from build123d import *

# Parameters (mm, degrees)
F0_W      = 12.5
F0_H      = 13.2
F1_DEPTH  = 6.5
F2_R      = 3.5
F3_DEPTH  = 5
F4_R      = 3
F5_DEPTH  = 10
F6_SIZE   = 0.5
F7_W      = 12.7
F7_H      = 1.5
F8_DEPTH  = 7
F10_DEPTH = 1


with BuildPart() as f1:
    # F0 (on Top) → F1 (new body)
    with BuildSketch(Plane.XY):
        Rectangle(F0_W, F0_H)
    extrude(amount=F1_DEPTH)

    # F2 (on face) → F3 (join)
    with BuildSketch(Plane.XY.offset(6.5)):
        Circle(F2_R)
    extrude(amount=F3_DEPTH)

    # F4 (on face) → F5 (join)
    with BuildSketch(Plane.XY.offset(11.5)):
        Circle(F4_R)
    extrude(amount=F5_DEPTH)

    # F6
    f6_edges = [f1.edges().sort_by_distance(p)[0] for p in [
        (-3, 0, 21.5),
    ]]
    chamfer(f6_edges, length=F6_SIZE)

    # F7 (on face) → F8 (cut)
    with BuildSketch(Plane.XY.offset(21.5)):
        with Locations((0, -2.25)):
            Rectangle(F7_W, F7_H)
    extrude(amount=-F8_DEPTH, mode=Mode.SUBTRACT)

    # F9 (on Front) → F10 (join, symmetric)
    with BuildSketch(Plane.XZ):
        Polygon((-6.25, 3.25), (-7, 3.25), (-7, -3.5), (-6.5, -3.5), (-6.5, 2.75), (-6.25, 2.75), align=None)
        Polygon((6.25, 2.75), (6.5, 2.75), (6.5, -3.5), (7, -3.5), (7, 3.25), (6.25, 3.25), align=None)
    extrude(amount=F10_DEPTH, both=True)


solid = f1.part
Geometry check sheet. Reference: the model listing, model coordinates, mm. A direction names the side the tool comes from. Round coordinates to 2 decimals unless told otherwise and drop trailing zeros. Loops run counter-clockwise (first coordinate to the right, second up) from the corner with the lowest first, then second, coordinate; pieces in that order, holes last. Notation, with made-up numbers: (31.25, 48.5) - (64.25, 48.5) arc R16 cw to (64.25, 77.5) - close; hole circle Ø10 at (48.25, -2.5). An arc over 180 degrees is marked (long way). One line per question, with ' | ' between items. Start each with the question number.
1. Tool access check on faces 5 (the face through (0, -2, 14.5)), 6 (the face through (0, 6.6, 3)), 7 (the face through (1.61, 2.53, 16.18)). Record the directions out of +Z, -Z, +X, -X, +Y, -Y that give a thin tool (end or side, any length) a straight path to the whole face; none if there is none.
2. Cross-section at D-D on z = 16.25. Record the cut outline in (x, y).
3. Cross-section at A-A on z = -1.25. Record the cut outline in (x, y), then the cut area to 3 significant figures.
4. Depth check by flat-ended pin: pin 1 (4 mm diameter, centred on x = -1.5, y = 0, fed in from -Z); pin 2 (0.8 mm diameter, centred on x = -7, y = 0, fed in from +Z); pin 3 (0.6 mm diameter, centred on x = -6.5, z = -1, fed in from -Y). Enter the tip coordinate at first touch or a pass-through.
5. Scan lines: line 1 (X direction, y = 1.5, z = 4.5); line 2 (Z direction, x = 6, y = -5); line 3 (Z direction, x = 1.25, y = 1.25). Record each from-to range of solid material in increasing order. Write a range as [from, to].
6. Draft check along X on faces 1 (the face through (-6.5, 0, 0)), 2 (the face through (0.082, 2.634, 21.365)), 3 (the face through (0, -6.6, 3)), 4 (the face through (6.5, 0, 0)). Enter one of: released by +X, released by -X, zero draft, split by the parting line, or undercut.
7. Cross-section at C-C on x = 0. Record the cut outline in (y, z), then the cut area to 3 significant figures.
8. Cross-section at B-B on y = 0. Record the cut outline in (x, z), then the cut area to 3 significant figures.
Taken from the geometry:
1) face 5: +Z, +X, -X, -Y | face 6: +Z, -Z, +X, -X, +Y | face 7: +Z
2) outline: (-2.6, -1.5) - (2.6, -1.5) arc R3 ccw (long way) to start
3) outline: (-7, -1) - (-6.5, -1) - (-6.5, 1) - (-7, 1) - close; (6.5, -1) - (7, -1) - (7, 1) - (6.5, 1) - close | area: 2.00 mm²
4) pin 1: z = 0 | pin 2: z = 3.25 | pin 3: y = -1
5) line 1: [-6.25, 6.25] | line 2: [0, 6.5] | line 3: [0, 21.5]
6) face 1: undercut | face 2: split by the parting line | face 3: zero draft | face 4: undercut
7) outline: (-6.6, 0) - (6.6, 0) - (6.6, 6.5) - (3.5, 6.5) - (3.5, 11.5) - (3, 11.5) - (3, 21) - (2.5, 21.5) - (-1.5, 21.5) - (-1.5, 14.5) - (-3, 14.5) - (-3, 11.5) - (-3.5, 11.5) - (-3.5, 6.5) - (-6.6, 6.5) - close | area: 170 mm²
8) outline: (-7, -3.5) - (-6.5, -3.5) - (-6.5, 2.75) - (-6.25, 2.75) - (-6.25, 0) - (6.25, 0) - (6.25, 2.75) - (6.5, 2.75) - (6.5, -3.5) - (7, -3.5) - (7, 3.25) - (6.25, 3.25) - (6.25, 6.5) - (3.5, 6.5) - (3.5, 11.5) - (3, 11.5) - (3, 21) - (2.5, 21.5) - (-2.5, 21.5) - (-3, 21) - (-3, 11.5) - (-3.5, 11.5) - (-3.5, 6.5) - (-6.25, 6.5) - (-6.25, 3.25) - (-7, 3.25) - close | area: 183 mm²
